```python
from build123d import *

# Parameters (mm, degrees)
SKETCH1_R           = 12.5
SKETCH1_R_2         = 3.25
BOSS_EXTRUDE1_DEPTH = 20
SKETCH2_R           = 6.5
CUT_EXTRUDE1_DEPTH  = 5
SKETCH3_R           = 6.5
CUT_EXTRUDE2_DEPTH  = 5


with BuildPart() as part:
    # Sketch1 → Boss-Extrude1 (new body)
    with BuildSketch(Plane(origin=(0, 0, 0), x_dir=(1, 0, 0), z_dir=(0, 1, 0))):
        Circle(SKETCH1_R)
        Circle(SKETCH1_R_2, mode=Mode.SUBTRACT)
    extrude(amount=BOSS_EXTRUDE1_DEPTH)

    # Sketch2 → Cut-Extrude1 (cut)
    with BuildSketch(Plane(origin=(0, 0, 0), x_dir=(1, 0, 0), z_dir=(0, 1, 0))):
        Circle(SKETCH2_R)
    extrude(amount=CUT_EXTRUDE1_DEPTH, mode=Mode.SUBTRACT)

    # Sketch3 → Cut-Extrude2 (cut)
    with BuildSketch(Plane(origin=(0, 20, 0), x_dir=(1, 0, 0), z_dir=(0, 1, 0))):
        Circle(SKETCH3_R)
    extrude(amount=-CUT_EXTRUDE2_DEPTH, mode=Mode.SUBTRACT)


solid = part.part
```
Check sheet for the modelled part. Datum: model origin and axes. Units: mm. A direction names the side the tool comes from. Round coordinates to 2 decimals unless told otherwise and drop trailing zeros. Order: outer loops, then holes, each group sorted by start corner. A loop starts at its lowest first (then second) coordinate and runs counter-clockwise, first axis right, second up. Notation, with made-up numbers: (35.25, -15) -> (87.25, -15) arc R16 cw to (87.25, 10) -> close; hole circle Ø10 at (84.25, 66). An arc over 180 degrees is marked (long way). One line per item, written item: value. Start each with the question number.
Q1. Mould release check, pull along Z, two halves, no side actions. Record for faces 1 (the face through (11.923, 9.86, -3.755)), 2 (the face through (5, 0, 5)), 3 (the face through (-5.158, 2.465, 3.955)), 4 (the face through (-2, 5, -3)): pulls with the +Z half, pulls with the -Z half, needs draft (parallel to the pull), parting line crosses it, or undercut.
Q2. Cross-section at C-C (y = 1.5). Record the boundary of the cut face in (x, z), and give its area (3 significant figures).
Q3. Cross-section at A-A (z = 0). Record the boundary of the cut face in (x, y), and give its area (3 significant figures).
Q4. Gauge pin test, flat ends, axial feed: pin 1 Ø11.5 at (x, z) = (0, 0) entering from -Y; pin 2 Ø3 at (x, z) = (-6.5, -2) entering from -Y; pin 3 Ø2 at (y, z) = (10.5, -8.5) entering from +X; pin 4 Ø3 at (y, z) = (15, -6.5) entering from -X. Record the tip position at first contact, or that the pin passes through.
Q5. Cross-section at D-D (x = -10). Record the boundary of the cut face in (y, z).
Q6. Cross-section at B-B (x = 0). Record the boundary of the cut face in (y, z).
Q7. Thickness scan on line 1 (Z direction, x = 0, y = 3); line 2 (Z direction, x = 0, y = 8). Record the ranges inside material, lowest first.
Q8. Set-up check for faces 5 (the face through (5, 20, 5)), 6 (the face through (-5.158, 17.535, 3.955)): record each of +Z, -Z, +X, -X, +Y, -Y from which the full face is reachable in a straight line by a thin tool's end or side.
Completed:
1. face 1: parting line crosses it
1. face 2: needs draft
1. face 3: undercut
1. face 4: undercut
2. outline: circle Ø25 at (0, 0); hole circle Ø13 at (0, 0)
2. area: 358 mm²
3. outline: (-12.5, 0) -> (-6.5, 0) -> (-6.5, 5) -> (-3.25, 5) -> (-3.25, 15) -> (-6.5, 15) -> (-6.5, 20) -> (-12.5, 20) -> close; (3.25, 5) -> (6.5, 5) -> (6.5, 0) -> (12.5, 0) -> (12.5, 20) -> (6.5, 20) -> (6.5, 15) -> (3.25, 15) -> close
3. area: 305 mm²
4. pin 1: stops at y = 5
4. pin 2: stops at y = 0
4. pin 3: stops at x = 10
4. pin 4: stops at x = -11.46
5. outline: (0, -7.5) -> (20, -7.5) -> (20, 7.5) -> (0, 7.5) -> close
6. outline: (0, -12.5) -> (20, -12.5) -> (20, -6.5) -> (15, -6.5) -> (15, -3.25) -> (5, -3.25) -> (5, -6.5) -> (0, -6.5) -> close; (0, 6.5) -> (5, 6.5) -> (5, 3.25) -> (15, 3.25) -> (15, 6.5) -> (20, 6.5) -> (20, 12.5) -> (0, 12.5) -> close
7. line 1: z = -12.5 to -6.5, 6.5 to 12.5
7. line 2: z = -12.5 to -3.25, 3.25 to 12.5
8. face 5: +Z, -Z, +X, -X, +Y
8. face 6: +Y
